Design review of the part built by this model. Coordinates are the model's own, in mm. A direction names the side the tool comes from. Coordinates: 2 decimals unless noted, no trailing zeros. Write each loop counter-clockwise with the first axis right and the second up, starting at its lowest first coordinate (ties: lowest second). Pieces come first, ordered by that corner, then holes. Notation, with made-up numbers: M 32,-37.5 L 56,-37.5 A9 cw 56,-32.5 Z; hole C 6,26.5 d9. An arc over 180 degrees is marked long. Write item = value, one per line.
```python
from build123d import *

# Parameters (mm, degrees)
SKETCH1_R           = 20
BOSS_EXTRUDE1_DEPTH = 18
SKETCH2_R           = 5
CUT_EXTRUDE1_DEPTH  = 10
SKETCH3_R           = 1.5
CUT_EXTRUDE2_DEPTH  = 8


with BuildPart() as part:
    # Sketch1 → Boss-Extrude1 (new body)
    with BuildSketch(Plane(origin=(0, 0, 0), x_dir=(1, 0, 0), z_dir=(0, 1, 0))):
        Circle(SKETCH1_R)
    extrude(amount=BOSS_EXTRUDE1_DEPTH)

    # Sketch2 → Cut-Extrude1 (cut)
    with BuildSketch(Plane(origin=(0, 18, 0), x_dir=(1, 0, 0), z_dir=(0, 1, 0))):
        Circle(SKETCH2_R)
    extrude(amount=-CUT_EXTRUDE1_DEPTH, mode=Mode.SUBTRACT)

    # Sketch3 → Cut-Extrude2 (cut)
    with BuildSketch(Plane.XZ):
        with Locations((11, -11)):
            Circle(SKETCH3_R)
        with Locations((-11, -11)):
            Circle(SKETCH3_R)
        with Locations((11, 11)):
            Circle(SKETCH3_R)
        with Locations((-11, 11)):
            Circle(SKETCH3_R)
    extrude(amount=-CUT_EXTRUDE2_DEPTH, mode=Mode.SUBTRACT)


solid = part.part
```
Q1. Machinability: for faces 1 (the cylindrical face through (-1.08, 13.07, 4.88)), 2 (the cylindrical face through (-12.2, 3.9, -11.9)), 3 (the flat face through (4, 18, 4)), which of the approach directions +Z, -Z, +X, -X, +Y, -Y give a long, thin tool a straight path to every point of the face, cutting with its end or side? Answer none if there is none.
Check result:
face_1 = +Y
face_2 = -Y
face_3 = +Z, -Z, +X, -X, +Y
Q2. Wall thickness on line 1 (Z direction, x = -11, y = 4); line 2 (X direction, y = 13, z = 0); line 3 (Z direction, x = 17.5, y = 6): over which ranges is each line inside the solid? List them lowest first.
Check result:
line_1 = -16.7 to -12.5, -9.5 to 9.5, 12.5 to 16.7
line_2 = -20 to -5, 5 to 20
line_3 = -9.68 to 9.68
Q3. The part is to be moulded in two halves that separate along Z. For faces 4 (the flat face through (11, 8, 11)), 5 (the cylindrical face through (-4.336, 8.874, 19.524)), 6 (the flat face through (0, 0, 0)), say which applies: +Z half, -Z half, draft (parallel to the pull), parting line (faces both ways), or undercut.
Check result:
face_4 = undercut
face_5 = parting line
face_6 = draft
Q4. Consider section A-A, the plane z = 0. State the section outline as (x, y) points, and give its area (3 significant figures).
Check result:
outline = M -20,0 L 20,0 L 20,18 L 5,18 L 5,8 L -5,8 L -5,18 L -20,18 Z
area = 620 mm²
Q5. Consider section B-B, the plane x = 0. State the section outline as (y, z) points, and give its area (3 significant figures).
Check result:
outline = M 0,-20 L 18,-20 L 18,-5 L 8,-5 L 8,5 L 18,5 L 18,20 L 0,20 Z
area = 620 mm²
Q6. Consider section C-C, the plane y = 6.5. State the section outline as (x, z) points, and give its area (3 significant figures).
Check result:
outline = C 0,0 d40; hole C -11,-11 d3; hole C -11,11 d3; hole C 11,-11 d3; hole C 11,11 d3
area = 1,230 mm²
Q7. Consider section D-D, the plane y = 13.25. State the section outline as (x, z) points.
Check result:
outline = C 0,0 d40; hole C 0,0 d10
Q8. For P1, Ø1.5, axis at y = 15.5, z = 11, coming from the +X side; P2, Ø2.5, axis at x = 11, z = 11, coming from the -Y side; P3, Ø3, axis at x = -2, z = 1, coming from the +Y side, all flat-tipped, find the tip position at first contact; note any pin that passes through.
Check result:
P1 = 17.17
P2 = 8
P3 = 8
